Source: CAD feature listing. Evaluate the final solid. Frame: model axes, mm. A direction names the side the tool comes from. Give positions to 0.01 mm unless a question says otherwise; leave off trailing zeros. Loops run counter-clockwise (first coordinate to the right, second up) from the corner with the lowest first, then second, coordinate; pieces in that order, holes last. Notation, with made-up numbers: M -36.5,70 L 2.5,70 A12 cw 2.5,92 Z; hole C 18,59 d10. An arc over 180 degrees is marked long. Put each result on its own line as item: value.
from build123d import *

# Parameters (mm, degrees)
F1_R           = 10.5
F2_DEPTH       = 12
F6_D           = 6.4
F6_CBORE_D     = 16
F6_CBORE_DEPTH = 8
F7_D           = 14
F9_D           = 3
F9_CBORE_D     = 4.9
F9_CBORE_DEPTH = 7


with BuildPart() as f2:
    # F1 (on offset) → F2 (new body)
    with BuildSketch(Plane.XY.offset(19)):
        with BuildLine():
            ThreePointArc((22, 30.3685692781), (0, 37.5), (-22, 30.3685692781))
            Line((-22, 30.3685692781), (-22, 5))
            ThreePointArc((-22, 5), (-23.4644660941, 1.4644660941), (-27, 0))
            Line((-27, 0), (-67.3498329619, 0))
            ThreePointArc((-67.3498329619, 0), (-43.1624837098, -38.8330753348), (0, -54))
            ThreePointArc((0, -54), (43.1624837098, -38.8330753348), (67.3498329619, 0))
            Line((67.3498329619, 0), (27, 0))
            ThreePointArc((27, 0), (23.4644660941, 1.4644660941), (22, 5))
            Line((22, 5), (22, 30.3685692781))
        make_face()
        Circle(F1_R, mode=Mode.SUBTRACT)
    extrude(amount=F2_DEPTH)

    # F6 (through all)
    with Locations(Plane.XY.offset(31)):
        with Locations((-13, 24), (13, 24), (-13, -24), (13, -24)):
            CounterBoreHole(F6_D / 2, F6_CBORE_D / 2, F6_CBORE_DEPTH)

    # F7 (through all)
    with Locations(Plane.XY.offset(31)):
        with Locations((-43.3012701892, -10), (43.3012701892, -10)):
            Hole(F7_D / 2)

    # F9 (through all)
    with Locations(Plane(origin=(0, 0, 19), x_dir=(1, 0, 0), z_dir=(0, 0, -1))):
        with Locations((0, 32), (0, -32)):
            CounterBoreHole(F9_D / 2, F9_CBORE_D / 2, F9_CBORE_DEPTH)


solid = f2.part
1. Material intervals for line 1 (Y direction, x = -7, z = 25.75); line 2 (Y direction, x = -13, z = 22.2); line 3 (X direction, y = -21, z = 27.75), sorted ascending. Write a range as from..to.
Found:
line 1: -53.64..-29.29, -18.71..-7.83, 7.83..18.71, 29.29..36.84
line 2: -52.76..-27.2, -20.8..20.8, 27.2..35.17
line 3: -58.86..-20.42, -5.58..5.58, 20.42..58.86
2. Section query A-A (z = 29.5). State how many separate pieces and enclosed holes the cut face has, plus the area to 3 significant figures.
Found:
separate pieces: 1
enclosed holes: 9
area: 5,510 mm^2
3. Section query C-C (y = -44). Output: boundary loops of the cut face in (x, z), plus the area to 3 significant figures.
Found:
outline: M -35.78,19 L 35.78,19 L 35.78,31 L -35.78,31 Z
area: 859 mm^2
4. Draft query along Y for faces 4 (the flat face through (-1, -18, 31)), 5 (the flat face through (12.9, -27.4, 23)), 6 (the flat face through (47, 0, 25)). Return one class per face: pulls with the +Y half, pulls with the -Y half, needs draft (parallel to the pull), parting line crosses it, or undercut.
Found:
face 4: needs draft
face 5: undercut
face 6: pulls with the +Y half
5. Contact query for flat-ended pins moving along their axis: P1, Ø6, axis at x = -13, y = 24, coming from the +Z side; P2, Ø1.5, axis at y = 12.5, z = 22, coming from the -X side; P3, Ø3, axis at y = 5.5, z = 23, coming from the +X side; P4, Ø7.5, axis at x = 13, y = 24, coming from the +Z side. Output: stop coordinate, or through.
Found:
P1: through
P2: x = -22
P3: x = 22.1
P4: z = 23
6. Section query B-B (x = -13). Output: boundary loops of the cut face in (y, z).
Found:
outline: M -52.76,19 L -27.2,19 L -27.2,23 L -32,23 L -32,31 L -52.76,31 Z; M -20.8,19 L 20.8,19 L 20.8,23 L 16,23 L 16,31 L -16,31 L -16,23 L -20.8,23 Z; M 27.2,19 L 35.17,19 L 35.17,31 L 32,31 L 32,23 L 27.2,23 Z
7. Section query D-D (x = 59). Output: boundary loops of the cut face in (y, z), plus the area to 3 significant figures.
Found:
outline: M -20.78,19 L 0,19 L 0,31 L -20.78,31 Z
area: 249 mm^2
8. Access query for faces 1 (the flat face through (22, 18, 25)), 2 (the cylindrical face through (11.959, 31.932, 27.056)), 3 (the flat face through (2, -32, 26)). Directions: +Z, -Z, +X, -X, +Y, -Y. A direction counts if a zero-diameter tool reaches every point of the face in a straight line with its end or side. Return the directions, or none.
Found:
face 1: +Z, -Z, +X, +Y
face 2: +Z
face 3: -Z
